Autodesk Inventor part; units mm, degrees
ref_plane "YZ Plane" through (0, 0, 0) normal (1, 0, 0) x (0, 1, 0)
ref_plane "XZ Plane" through (0, 0, 0) normal (0, 1, 0) x (-1, 0, 0)
ref_plane "XY Plane" through (0, 0, 0) normal (0, 0, 1) x (1, 0, 0)
sketch "Sketch1" plane through (0, 0, 0) normal (0, 0, 1) x (1, 0, 0)
  circle A0 centre (0, 0) radius 45
  circle A1 centre (70, 0) radius 30
  circle A2 centre (111, 0) radius 17.5
  circle A3 centre (138, 0) radius 9
  circle A4 centre (-70, 0) radius 30
  circle A5 centre (-111, 0) radius 17.5
  circle A6 centre (-138, 0) radius 9
  line L0 (-11.1486, 43.5971) -> (-115.3356, 16.9544)
  line L1 (11.1486, 43.5971) -> (115.3356, 16.9544)
  line L2 (-116.5093, 16.6102) -> (-140.8333, 8.5424)
  line L3 (116.5093, 16.6102) -> (140.8333, 8.5424)
  line L4 (-11.1486, -43.5971) -> (-115.3356, -16.9544)
  line L5 (11.1486, -43.5971) -> (115.3356, -16.9544)
  line L6 (140.8333, -8.5424) -> (116.5093, -16.6102)
  line L7 (-140.8333, -8.5424) -> (-116.5093, -16.6102)
  circle A7 centre (-138, 0) radius 1.5
  circle A8 centre (-111, 0) radius 3
  circle A9 centre (-70, 0) radius 3
  circle A10 centre (0, 0) radius 3
  circle A11 centre (70, 0) radius 3
  circle A12 centre (111, 0) radius 3
  circle A13 centre (138, 0) radius 1.5
  line L8 (-123.0921, -97.5699) -> (-152.3126, 20.9991) construction
  line L9 (-152.3126, 20.9991) -> (130.841, 90.7804) construction
  line L10 (130.841, 90.7804) -> (160.0615, -27.7887) construction
  line L11 (160.0615, -27.7887) -> (-123.0921, -97.5699) construction
  circle A14 centre (-41.1855, -28.1747) radius 1.5
  circle A15 centre (-41.1855, 28.1747) radius 1.5
  circle A16 centre (41.1855, 28.1747) radius 1.5
  circle A17 centre (41.1855, -28.1747) radius 1.5
  line L12 (0, 45) -> (0, -45)
  line L13 (-37.7402, 24.5088) -> (37.7402, -24.5088)
  line L14 (-37.7402, -24.5088) -> (37.7402, 24.5088)
  line L15 (-45, 0) -> (45, 0)
  point P0 (-88.1111, 23.9163)
  point P1 (-88.1111, -23.9163)
  point P2 (-65.5931, -29.6746)
  point P3 (65.5931, -29.6746)
  point P4 (88.1111, -23.9163)
  point P5 (88.1111, 23.9163)
  point P6 (65.5931, 29.6746)
  point P7 (-65.5931, 29.6746)
  point P8 (0, 0)
  dimension "d0" = 90
  dimension "d1" = 60
  dimension "d2" = 70
  dimension "d3" = 35
  dimension "d4" = 41
  dimension "d5" = 18
  dimension "d6" = 27
  dimension "d7" = 0
  dimension "d8" = 0
  dimension "d9" = 0
  dimension "d10" = 60
  dimension "d11" = 35
  dimension "d12" = 41
  dimension "d13" = 18
  dimension "d16" = 70
  dimension "d17" = 0
  dimension "d18" = 0
  dimension "d19" = 0
  dimension "d20" = 27
  dimension "d23" = 6
  dimension "d24" = 6
  dimension "d25" = 6
  dimension "d26" = 3
  dimension "d27" = 6
  dimension "d28" = 6
  dimension "d29" = 3
  dimension "d109" = 0.5
  dimension "d121" = 7.5
  dimension "d133" = 3
  dimension "d138" = 8.8
  dimension "d139" = 3.4005
  dimension "d140" = 3
  dimension "d141" = 3
  dimension "d142" = 3
  dimension "d143" = 7.5
  dimension "d145" = 8.8
  dimension "d146" = 7.5
  dimension "d148" = 8.8
  dimension "d151" = 8.8
  dimension "d152" = 3.4005
  dimension "d153" = 3.4005
  dimension "d155" = 7.5
  dimension "d156" = 3.4005
  dimension "d157" = 57
  dimension "d159" = 57
extrude "Extrusion1" add sketch "Sketch1" along normal blind 3 contours L14 A10 L12 A0 | A0 L1 A1 | A0 A1 L15 A10 L14 | A1 L1 A2 L5 A0 | A0 L15 A1 | L12 A10 L13 A0 | A1 L1 | A0 A1 L15 | A1 A0 L13 A10 L15 | A0 A4 L0 | L1 A2 A1 | A1 L5 A0 | L13 A0 L12 A10 | A10 L15 A4 A0 L13 | L12 A0 L14 A10 | L14 A0 A4 L15 A10 | L0 A4 | A4 A0 L4 A5 L0 | A2 A1 | A1 A2 | L5 A1 | A0 L4 A4 | L15 A0 A4 | A4 A0 L15 | A4 A5 L0 | A2 L5 A1 | L3 A3 L6 A2 | A5 A4 | A4 A5 | A3 | A4 L4 | A4 L4 A5 | A5 L7 A6 L2 | A6
equation "\"BendRadius\" = Thickness"
equation "\"BendReliefWidth\" = Thickness"
equation "\"BendReliefDepth\" = 0.5 * Thickness"
equation "\"CornerReliefSize\" = 4 * Thickness"
equation "\"MinimumRemnant\" = 2 * Thickness"
equation "\"TransitionRadius\" = BendRadius"
equation "\"JacobiRadiusSize\" = BendRadius"
equation "\"GapSize\" = Thickness"
properties part number "frame" material "PMMA Plastic"
Verification items for the finished model (mm, model axes). Give positions to 0.01 mm unless a question says otherwise; leave off trailing zeros. Write each loop counter-clockwise with the first axis right and the second up, starting at its lowest first coordinate (ties: lowest second). Pieces come first, ordered by that corner, then holes.
(1) Cross-section at B-B (x = 0). Enter the section's corners in (y, z), plus the area to 3 significant figures.
(2) Mould release check, pull along X, two halves, no side actions. Record for faces 1 (the face through (-72.4, 1.8, 1.5)), 2 (the face through (-2, -9, 3)), 3 (the face through (-101.533, 20.484, 1.479)), 4 (the face through (-77.594, 29.023, 1.479)): +X half, -X half, draft (parallel to the pull), parting line (faces both ways), or undercut.
(3) Material ranges on line 1 (Y direction, x = 0, z = 0.9); line 2 (X direction, y = -27.5, z = 1.15); line 3 (Y direction, x = 2, z = 0.3), recorded low to high.
(4) Gauge pin test, flat ends, axial feed: pin 1 (12 mm diameter, centred on x = 106.5, y = -13.5, fed in from -Z); pin 2 (1 mm diameter, centred on y = 7, z = 2, fed in from -X). Record the tip position at first contact, or that the pin passes through.
(5) Cross-section at A-A (x = -70). Enter the section's corners in (y, z).
(6) Cross-section at C-C (z = 2.4). State how many separate pieces and enclosed holes the cut face has, plus the area to 3 significant figures.
(7) Cross-section at D-D (y = 14). Enter the section's corners in (x, z), plus the area to 3 significant figures.
Worked out:
1. outline: (-45, 0) - (-3, 0) - (-3, 3) - (-45, 3) - close; (3, 0) - (45, 0) - (45, 3) - (3, 3) - close
1. area: 252 mm2
2. face 1: undercut
2. face 2: draft
2. face 3: -X half
2. face 4: undercut
3. line 1: y = -45 to -3, 3 to 45
3. line 2: x = -81.99 to -42.53, -39.85 to 39.85, 42.53 to 81.99
3. line 3: y = -44.96 to -2.24, 2.24 to 44.96
4. pin 1: stops at z = 0
4. pin 2: stops at x = -144.22
5. outline: (-30, 0) - (-3, 0) - (-3, 3) - (-30, 3) - close; (3, 0) - (30, 0) - (30, 3) - (3, 3) - close
6. separate pieces: 1
6. enclosed holes: 11
6. area: 16,000 mm2
7. outline: (-124.38, 0) - (124.38, 0) - (124.38, 3) - (-124.38, 3) - close
7. area: 746 mm2
